For this review, take the finished solid that the model builds, in its own axes (mm). A direction names the side the tool comes from. Round coordinates to 2 decimals unless told otherwise and drop trailing zeros. Order: outer loops, then holes, each group sorted by start corner. A loop starts at its lowest first (then second) coordinate and runs counter-clockwise, first axis right, second up. Notation, with made-up numbers: (-22.75, 65.5) - (-1.75, 65.5) arc R17 cw to (-1.75, 73.5) - close; hole circle Ø5 at (5, 7.25). An arc over 180 degrees is marked (long way). One line per question, with ' | ' between items.
```python
from build123d import *

# Parameters (mm, degrees)
EXTRUDE_1_DEPTH     = 6
SKETCH_2_R          = 1.25
CUT_EXTRUDE_1_DEPTH = 10
SKETCH_3_R          = 1.05
CUT_EXTRUDE_2_DEPTH = 81.845531726
SKETCH_4_R          = 2.55
CUT_EXTRUDE_3_DEPTH = 81.845531783
FILLET_1_R          = 2.1
SKETCH_5_W          = 8
SKETCH_5_H          = 6
EXTRUDE_2_DEPTH     = 20
FILLET_2_R          = 10
FILLET_3_R          = 10
SKETCH_7_R          = 1.55
EXTRUDE_3_DEPTH     = 6
FILLET_4_R          = 8


with BuildPart() as part:
    # ｽｹｯﾁ1 → ﾎﾞｽ - 押し出し1 (new body)
    with BuildSketch(Plane(origin=(0, 0, 0), x_dir=(1, 0, 0), z_dir=(0, 1, 0))):
        Polygon((0, -70), (0, 70), (36.5, 70), (36.5, 61), (40, 61), (40, 45), (20, 45), (20, -45), (40, -45), (40, -61), (36.5, -61), (36.5, -70), align=None)
    extrude(amount=EXTRUDE_1_DEPTH)

    # ｽｹｯﾁ2 → ｶｯﾄ - 押し出し1 (cut)
    with BuildSketch(Plane(origin=(40, 0, 0), x_dir=(0, 0, -1), z_dir=(1, 0, 0))):
        with Locations((48, 3)):
            Circle(SKETCH_2_R)
        with Locations((58, 3)):
            Circle(SKETCH_2_R)
        with Locations(Location((-48, 3, 0), (0, 0, 180))):
            Circle(SKETCH_2_R)
        with Locations(Location((-58, 3, 0), (0, 0, 180))):
            Circle(SKETCH_2_R)
    extrude(amount=-CUT_EXTRUDE_1_DEPTH, mode=Mode.SUBTRACT)

    # ｽｹｯﾁ3 → ｶｯﾄ - 押し出し2 (cut, through all)
    with BuildSketch(Plane(origin=(0, 6, 0), x_dir=(1, 0, 0), z_dir=(0, 1, 0))):
        with Locations((40.7, 58)):
            Circle(SKETCH_3_R)
        with Locations((40.7, 48)):
            Circle(SKETCH_3_R)
        with Locations((40.7, -48)):
            Circle(SKETCH_3_R)
        with Locations((40.7, -58)):
            Circle(SKETCH_3_R)
    extrude(amount=-CUT_EXTRUDE_2_DEPTH, mode=Mode.SUBTRACT)

    # ｽｹｯﾁ4 → ｶｯﾄ - 押し出し3 (cut, through all)
    with BuildSketch(Plane(origin=(0, 6, 0), x_dir=(1, 0, 0), z_dir=(0, 1, 0))):
        with Locations(Location((10, 0, 0), (0, 0, 270))):
            Circle(SKETCH_4_R)
        with Locations(Location((10, 60, 0), (0, 0, 270))):
            Circle(SKETCH_4_R)
        with Locations(Location((10, -60, 0), (0, 0, 270))):
            Circle(SKETCH_4_R)
    extrude(amount=-CUT_EXTRUDE_3_DEPTH, mode=Mode.SUBTRACT)

    # ﾌｨﾚｯﾄ1
    fillet_1_edges = [part.edges().sort_by_distance(p)[0] for p in [
        (36.5, 3, -61),
        (20, 3, -45),
        (20, 3, 45),
        (36.5, 3, 61),
    ]]
    fillet(fillet_1_edges, radius=FILLET_1_R)

    # ｽｹｯﾁ5 → ﾎﾞｽ - 押し出し2 (add)
    with BuildSketch(Plane(origin=(20, 0, 0), x_dir=(0, 0, -1), z_dir=(1, 0, 0))):
        with Locations((0, 3)):
            Rectangle(SKETCH_5_W, SKETCH_5_H)
    extrude(amount=EXTRUDE_2_DEPTH)

    # ﾌｨﾚｯﾄ2
    fillet_2_edges = [part.edges().sort_by_distance(p)[0] for p in [
        (20, 3, 4),
        (20, 3, -4),
    ]]
    fillet(fillet_2_edges, radius=FILLET_2_R)

    # ﾌｨﾚｯﾄ3
    fillet_3_edges = [part.edges().sort_by_distance(p)[0] for p in [
        (0, 3, 70),
        (0, 3, -70),
    ]]
    fillet(fillet_3_edges, radius=FILLET_3_R)

    # ｽｹｯﾁ7 → ﾎﾞｽ - 押し出し3 (add, through all)
    # profile 1 of 2: a face of its own
    with BuildSketch(Plane(origin=(0, 6, 0), x_dir=(1, 0, 0), z_dir=(0, 1, 0))):
        with BuildLine():
            Line((23.5, 28.25), (20, 28.25))
            Line((20, 28.25), (20, 21.75))
            Line((20, 21.75), (23.5, 21.75))
            ThreePointArc((23.5, 21.75), (26.75, 25), (23.5, 28.25))
        make_face()
        with Locations(Location((23.5, 25, 0), (0, 0, 270))):
            Circle(SKETCH_7_R, mode=Mode.SUBTRACT)
    # profile 2 of 2: a face of its own
    with BuildSketch(Plane(origin=(0, 6, 0), x_dir=(1, 0, 0), z_dir=(0, 1, 0))):
        with BuildLine():
            Line((20, -21.75), (23.5, -21.75))
            ThreePointArc((23.5, -21.75), (26.75, -25), (23.5, -28.25))
            Line((23.5, -28.25), (20, -28.25))
            Line((20, -28.25), (20, -21.75))
        make_face()
        with Locations(Location((23.5, -25, 0), (0, 0, 90))):
            Circle(SKETCH_7_R, mode=Mode.SUBTRACT)
    extrude(amount=-EXTRUDE_3_DEPTH)

    # ﾌｨﾚｯﾄ4
    fillet_4_edges = [part.edges().sort_by_distance(p)[0] for p in [
        (20, 3, 28.25),
        (20, 3, 21.75),
        (20, 3, -28.25),
        (20, 3, -21.75),
    ]]
    fillet(fillet_4_edges, radius=FILLET_4_R)


solid = part.part
```
(1) For probe 1 along X at (y, z) = (1.5, -60); probe 2 along Y at (x, z) = (33.75, 58); probe 3 along Z at (x, y) = (26.5, 5), list the stretches that pass through material, from the lowest coordinate up. Write a range as [from, to].
Output values:
probe 1: [0, 7.45], [12.55, 40] | probe 2: [0, 1.75], [4.25, 6] | probe 3: [-70, -45], [-26.25, -23.75], [-4.63, 4.63], [23.75, 26.25], [45, 70]
(2) We need section B-B on z = -25. State the section outline as (x, y) points.
Output values:
outline: (0, 0) - (21.95, 0) - (21.95, 6) - (0, 6) - close; (25.05, 0) - (26.75, 0) - (26.75, 6) - (25.05, 6) - close
(3) We need section A-A on x = 32. State the section outline as (y, z) points.
Output values:
outline: (0, -70) - (6, -70) - (6, -45) - (0, -45) - close; (0, -4) - (6, -4) - (6, 4) - (0, 4) - close; (0, 45) - (6, 45) - (6, 70) - (0, 70) - close; hole circle Ø2.5 at (3, -58); hole circle Ø2.5 at (3, -48); hole circle Ø2.5 at (3, 48); hole circle Ø2.5 at (3, 58)
(4) Mouldability with a two-part tool opening along Y and no side actions: class faces 4 (the flat face through (16, 0, -1)), 5 (the cylindrical face through (35.07, 3.38, -59.19)), 6 (the flat face through (40, 3, 53)) as released by +Y, released by -Y, zero draft, split by the parting line, or undercut.
Output values:
face 4: released by -Y | face 5: undercut | face 6: zero draft
(5) For faces 1 (the flat face through (31, 3, 45)), 2 (the flat face through (36.5, 3, 67)), 3 (the cylindrical face through (35.07, 3.05, -46.75)), list the 3-axis set-ups (+Z, -Z, +X, -X, +Y, -Y) from which the entire face can be reached by the end or side of a thin tool; tool diameter is ignored.
Output values:
face 1: +X, +Y, -Y | face 2: +Z, +X, +Y, -Y | face 3: +X
(6) Insertion check: pin 1 (2 mm diameter, centred on y = 4, z = 36, fed in from +X); pin 2 (1.5 mm diameter, centred on x = 39.5, y = 4, fed in from +Z); pin 3 (0.8 mm diameter, centred on y = 3, z = -58, fed in from +X); pin 4 (4 mm diameter, centred on x = 10, z = -60, fed in from +Y). Each pin has a flat end and moves straight along its axis. Give the tip position at first contact, or say it passes through.
Output values:
pin 1: x = 20.01 | pin 2: z = 61 | pin 3: x = 30 | pin 4: through
(7) We need section D-D on x = 4.5. State the section outline as (y, z) points.
Output values:
outline: (0, -68.35) - (6, -68.35) - (6, 68.35) - (0, 68.35) - close
(8) We need section C-C on z = 0. State the section outline as (x, y) points, plus the area to 3 significant figures.
Output values:
outline: (0, 0) - (7.45, 0) - (7.45, 6) - (0, 6) - close; (12.55, 0) - (40, 0) - (40, 6) - (12.55, 6) - close | area: 209 mm^2
